Design review of the part built by this model. Coordinates are the model's own, in mm. A direction names the side the tool comes from. Round coordinates to 2 decimals unless told otherwise and drop trailing zeros. Order: outer loops, then holes, each group sorted by start corner. A loop starts at its lowest first (then second) coordinate and runs counter-clockwise, first axis right, second up. Notation, with made-up numbers: (41.25, 10.25) - (56.25, 10.25) arc R25 cw to (56.25, 46.25) - close; hole circle Ø3 at (7.25, 60). An arc over 180 degrees is marked (long way). Use CSV: the item, a comma, the result in double quotes. Start each with the question number.
from build123d import *

# Parameters (mm, degrees)
SKETCH_1_R          = 6
EXTRUDE_1_DEPTH     = 7
SKETCH_2_R          = 9
EXTRUDE_2_DEPTH     = 1
SKETCH_3_R          = 9
EXTRUDE_3_DEPTH     = 1
SKETCH_4_R          = 1.5
CUT_EXTRUDE_2_DEPTH = 11
SKETCH_5_R          = 5
SKETCH_5_R_2        = 2
CUT_EXTRUDE_3_DEPTH = 0.5
SKETCH_6_R          = 5
SKETCH_6_R_2        = 2
CUT_EXTRUDE_4_DEPTH = 0.5


with BuildPart() as part:
    # 草图1 → 凸台-拉伸1 (new body)
    with BuildSketch(Plane.XY):
        Circle(SKETCH_1_R)
    extrude(amount=EXTRUDE_1_DEPTH)

    # 草图2 → 凸台-拉伸2 (add)
    with BuildSketch(Plane.XY.offset(7)):
        Circle(SKETCH_2_R)
    extrude(amount=EXTRUDE_2_DEPTH)

    # 草图3 → 凸台-拉伸3 (add)
    with BuildSketch(Plane(origin=(0, 0, 0), x_dir=(-1, 0, 0), z_dir=(0, 0, -1))):
        Circle(SKETCH_3_R)
    extrude(amount=EXTRUDE_3_DEPTH)

    # 草图4 → 切除-拉伸2 (cut)
    with BuildSketch(Plane.XY.offset(8)):
        Circle(SKETCH_4_R)
    extrude(amount=-CUT_EXTRUDE_2_DEPTH, mode=Mode.SUBTRACT)

    # 草图5 → 切除-拉伸3 (cut)
    with BuildSketch(Plane(origin=(0, 0, -1), x_dir=(-1, 0, 0), z_dir=(0, 0, -1))):
        Circle(SKETCH_5_R)
        Circle(SKETCH_5_R_2, mode=Mode.SUBTRACT)
    extrude(amount=-CUT_EXTRUDE_3_DEPTH, mode=Mode.SUBTRACT)

    # 草图6 → 切除-拉伸4 (cut)
    with BuildSketch(Plane.XY.offset(8)):
        Circle(SKETCH_6_R)
        Circle(SKETCH_6_R_2, mode=Mode.SUBTRACT)
    extrude(amount=-CUT_EXTRUDE_4_DEPTH, mode=Mode.SUBTRACT)


solid = part.part
Q1. For L1, parallel to Y at x = 0, z = 7.7; L2, parallel to Z at x = -6.5, y = 3; L3, parallel to Z at x = 0.25, y = -4.5, list the stretches that pass through material, from the lowest coordinate up. Write a range as [from, to].
Q2. Take a section at D-D (z = 4.25). State the section outline as (x, y) points.
Q3. Take a section at C-C (y = 5.75). State the section outline as (x, z) points.
Q4. Tool access review of faces 5 (the cylindrical face through (-1.172, 8.923, 7.493)), 6 (the flat face through (-0.1, -2.2, 7.5)), 7 (the flat face through (-4, -4, -1)), 8 (the flat face through (0.1, -2.2, -0.5)), 9 (the flat face through (2, -6, 7)): name each direction out of +Z, -Z, +X, -X, +Y, -Y from which nothing blocks a thin tool from reaching the whole face with its end or side.
Q5. The part is to be moulded in two halves that separate along Y. For faces 1 (the cylindrical face through (-6, 0, 3)), 2 (the flat face through (-2, -6, 0)), 3 (the cylindrical face through (1.08, -4.88, -0.75)), 4 (the cylindrical face through (0.434, -1.952, -0.754)), say which applies: +Y half, -Y half, draft (parallel to the pull), parting line (faces both ways), or undercut.
Q6. Clearance check with flat-ended pins moving along their axes: pin 1 (1 mm diameter, centred on x = 4.5, z = 1, fed in from -Y); pin 2 (1.5 mm diameter, centred on y = -4.5, z = 3, fed in from +X); pin 3 (1.5 mm diameter, centred on x = -6, z = 6, fed in from -Y). State where each tip first meets the part, or that it passes through.
Findings below:
1,L1,"y = [-9, -5], [-2, -1.5], [1.5, 2], [5, 9]"
1,L2,"z = [-1, 0], [7, 8]"
1,L3,"z = [-0.5, 7.5]"
2,outline,"circle Ø12 at (0, 0); hole circle Ø3 at (0, 0)"
3,outline,"(-6.92, -1) - (6.92, -1) - (6.92, 0) - (1.71, 0) - (1.71, 7) - (6.92, 7) - (6.92, 8) - (-6.92, 8) - (-6.92, 7) - (-1.71, 7) - (-1.71, 0) - (-6.92, 0) - close"
4,face 5,"+Z, -Z"
4,face 6,"+Z"
4,face 7,"-Z, +X, -X, +Y, -Y"
4,face 8,"-Z"
4,face 9,"none"
5,face 1,"parting line"
5,face 2,"draft"
5,face 3,"undercut"
5,face 4,"undercut"
6,pin 1,"stops at y = -4.47"
6,pin 2,"stops at x = 4.68"
6,pin 3,"stops at y = -2.9"
